Part model, mm, in its own coordinate system. Face numbers are marked on the shaded views. A direction names the side the tool comes from. Coordinates: 2 decimals unless noted, no trailing zeros. Write each loop counter-clockwise with the first axis right and the second up, starting at its lowest first coordinate (ties: lowest second). Pieces come first, ordered by that corner, then holes. Notation, with made-up numbers: (49.25, 44.25) -> (74.25, 44.25) arc R29 ccw to (74.25, 68.25) -> close; hole circle Ø2 at (70, -22.5). An arc over 180 degrees is marked (long way). Write item = value, one per line.
from build123d import *

# Parameters (mm, degrees)
SKETCH1_R           = 2.25
SKETCH1_R_2         = 1.3
BOSS_EXTRUDE1_DEPTH = 6.35
FILLET1_R           = 2


with BuildPart() as part:
    # Sketch1 → Boss-Extrude1 (new body)
    with BuildSketch(Plane.XY):
        Polygon((0, 0), (0, 27.94), (15.748, 27.94), (15.748, 5), (25.748, 5), (25.748, 0), (25.748, -15), (0, -15), align=None)
        with Locations((20.748, -5)):
            Circle(SKETCH1_R, mode=Mode.SUBTRACT)
        with Locations((2.54, 25.4)):
            Circle(SKETCH1_R_2, mode=Mode.SUBTRACT)
        with Locations((13.208, 2.54)):
            Circle(SKETCH1_R_2, mode=Mode.SUBTRACT)
    extrude(amount=BOSS_EXTRUDE1_DEPTH)

    # Fillet1
    fillet1_edges = [part.edges().sort_by_distance(p)[0] for p in [
        (0, 27.94, 3.175),
        (15.748, 27.94, 3.175),
        (15.748, 5, 3.175),
        (25.748, 5, 3.175),
        (25.748, -15, 3.175),
        (0, -15, 3.175),
    ]]
    fillet(fillet1_edges, radius=FILLET1_R)


solid = part.part
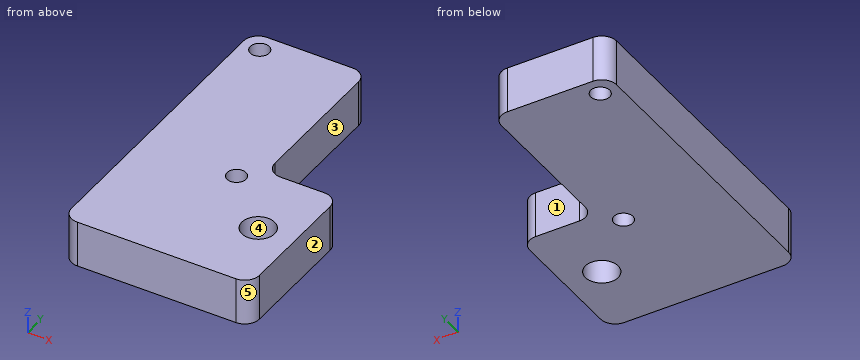
Q1. Saw through at C-C on z = 2. Give the cut face in (x, y), and give its area (3 significant figures).
Model answer:
outline = (0, -13) arc R2 ccw to (2, -15) -> (23.75, -15) arc R2 ccw to (25.75, -13) -> (25.75, 3) arc R2 ccw to (23.75, 5) -> (17.75, 5) arc R2 cw to (15.75, 7) -> (15.75, 25.94) arc R2 ccw to (13.75, 27.94) -> (2, 27.94) arc R2 ccw to (0, 25.94) -> close; hole circle Ø2.6 at (2.54, 25.4); hole circle Ø2.6 at (13.21, 2.54); hole circle Ø4.5 at (20.75, -5)
area = 846 mm²
Q2. Pin check, flat tips, straight feed: pin 1 (1.6 mm diameter, centred on x = 13.208, y = 2.54, fed in from +Z); pin 2 (3 mm diameter, centred on y = 12, z = 2, fed in from +X). Stop position of each tip, or through.
Model answer:
pin_1 = through
pin_2 = 15.75
Q3. Saw through at D-D on y = 21.5. Give the cut face in (x, z), and give its area (4 significant figures).
Model answer:
outline = (0, 0) -> (15.75, 0) -> (15.75, 6.35) -> (0, 6.35) -> close
area = 100.0 mm²
Q4. Which spindle directions (+Z, -Z, +X, -X, +Y, -Y) get a long thin tool onto all of the face, cutting with end or side? Do the marked faces 1 and 2. Say none if no direction does.
Model answer:
face_1 = +Z, -Z, +X, +Y
face_2 = +Z, -Z, +X, +Y, -Y
Q5. Mould opens along Y. For the marked faces 3, 4 and 5 say: released by +Y, released by -Y, zero draft, split by the parting line, or undercut.
Model answer:
face_3 = zero draft
face_4 = undercut
face_5 = released by -Y
Q6. Saw through at B-B on x = 2.54. Give the cut face in (y, z).
Model answer:
outline = (-15, 0) -> (24.1, 0) -> (24.1, 6.35) -> (-15, 6.35) -> close; (26.7, 0) -> (27.94, 0) -> (27.94, 6.35) -> (26.7, 6.35) -> close
Q7. Saw through at A-A on y = 2.54. Give the cut face in (x, z).
Model answer:
outline = (0, 0) -> (11.91, 0) -> (11.91, 6.35) -> (0, 6.35) -> close; (14.51, 0) -> (25.75, 0) -> (25.75, 6.35) -> (14.51, 6.35) -> close
Q8. Probe line 1 (Y direction, x = 2.54, z = 2.25); line 2 (X direction, y = 1.5, z = 5.25); line 3 (X direction, y = -6, z = 5). List the from-to ranges inside material, lowest first. Write a range as from..to.
Model answer:
line_1 = -15..24.1, 26.7..27.94
line_2 = 0..12.43, 13.99..25.75
line_3 = 0..18.73, 22.76..25.75
